Build history of the part. All positions in model axes, mm. A direction names the side the tool comes from. Give positions to 0.01 mm unless a question says otherwise; leave off trailing zeros. Order: outer loops, then holes, each group sorted by start corner. A loop starts at its lowest first (then second) coordinate and runs counter-clockwise, first axis right, second up. Notation, with made-up numbers: (25.25, -13) -> (68.25, -13) arc R31 cw to (68.25, 16) -> close; hole circle Ø3 at (46.5, -31.5). An arc over 180 degrees is marked (long way). One line per question, with ' | ' between items. Start each with the question number.
(1) Drill centre lines: L1, parallel to Y at x = 0, z = 2 (3 decimals); L2, parallel to X at y = 3.5, z = 5.75; L3, parallel to X at y = -6, z = 3.75. Where is each one in solid material? Low to high. Write a range as from..to.
(2) Pull direction X, two halves, no side cores. Call faces 4 (the face through (17, -10.376, 3)), 5 (the face through (48.018, 7.826, 3.451)), 6 (the face through (17, 10.254, 3)), 7 (the face through (34, -15.875, 3)): +X half, -X half, draft (parallel to the pull), parting line (faces both ways), or undercut.
(3) Cut at A-A (x = 0). Give the cut face in (y, z) (3 decimals), then the cut area to 4 significant figures.
(4) Cut at B-B (z = 1.5). Give the cut face in (x, y) (3 decimals), then the cut area to 3 significant figures.
(5) Which spindle directions (+Z, -Z, +X, -X, +Y, -Y) get a long thin tool onto all of the face, cutting with end or side? Do faces 1 (the face through (-17, 10.376, 3)), 2 (the face through (-17, -10.376, 3)), 3 (the face through (47.89, -8.05, 3.45)). Say none if no direction does.
(6) Pin check, flat tips, straight feed: pin 1 Ø3.5 at (x, z) = (-14.5, 4.5) entering from -Y; pin 2 Ø3.5 at (x, z) = (16, 4.5) entering from +Y; pin 3 Ø2 at (x, z) = (-16, 3) entering from +Y; pin 4 Ø10 at (x, y) = (-29, 0) entering from -Z. Stop position of each tip, or through.
(7) Cut at D-D (y = -12). Give the cut face in (x, z).
(8) Cut at C-C (y = 1). Give the cut face in (x, z), then the cut area to 3 significant figures.
from build123d import *

# Parameters (mm, degrees)
F0_R     = 11
F1_DEPTH = 7


with BuildPart() as f1:
    # F0 (on Top) → F1 (new body)
    with BuildSketch(Plane.XY):
        Polygon((-21.865436, -10.375739), (-15.875, 0), (-21.865436, 10.375739), (-25.040436, 15.875), (-43.371307, 15.875), (-52.536742, 0), (-43.371307, -15.875), (-25.040436, -15.875), align=None)
        with Locations((-34.205871, 0)):
            Circle(F0_R, mode=Mode.SUBTRACT)
        with BuildLine():
            ThreePointArc((-12.014977, 10.375739), (-14.878733, 5.535245), (-15.875, 0))
            ThreePointArc((-15.875, 0), (-14.878733, -5.535245), (-12.014977, -10.375739))
            ThreePointArc((-12.014977, -10.375739), (0, -15.875), (12.014977, -10.375739))
            ThreePointArc((12.014977, -10.375739), (14.878733, -5.535245), (15.875, 0))
            ThreePointArc((15.875, 0), (14.906507, 5.460006), (12.1192, 10.25381))
            ThreePointArc((12.1192, 10.25381), (0.080201, 15.874797), (-12.014977, 10.375739))
        make_face()
        Circle(F0_R, mode=Mode.SUBTRACT)
        with BuildLine():
            Line((-21.865436, 10.375739), (-15.875, 0))
            ThreePointArc((-15.875, 0), (-14.878733, 5.535245), (-12.014977, 10.375739))
            Line((-12.014977, 10.375739), (-21.865436, 10.375739))
        make_face()
        with BuildLine():
            ThreePointArc((-12.014977, -10.375739), (-14.878733, -5.535245), (-15.875, 0))
            Line((-15.875, 0), (-21.865436, -10.375739))
            Line((-21.865436, -10.375739), (-12.014977, -10.375739))
        make_face()
        with BuildLine():
            ThreePointArc((15.875, 0), (14.878733, -5.535245), (12.014977, -10.375739))
            Line((12.014977, -10.375739), (21.865436, -10.375739))
            Line((21.865436, -10.375739), (15.875, 0))
        make_face()
        with BuildLine():
            Line((21.79504, 10.25381), (12.1192, 10.25381))
            ThreePointArc((12.1192, 10.25381), (14.906507, 5.460006), (15.875, 0))
            Line((15.875, 0), (21.79504, 10.25381))
        make_face()
        Polygon((21.79504, 10.25381), (15.875, 0), (21.865436, -10.375739), (25.040436, -15.875), (43.371307, -15.875), (52.536742, 0), (43.371307, 15.875), (25.040436, 15.875), align=None)
        with Locations((34.205871, 0)):
            Circle(F0_R, mode=Mode.SUBTRACT)
    extrude(amount=F1_DEPTH)


solid = f1.part
Result set:
1) L1: y = -15.875..-11, 11..15.875 | L2: x = -50.52..-44.63, -23.78..-10.43, 10.43..23.78, 44.63..50.52 | L3: x = -49.07..-43.43, -24.99..-9.22, 9.22..24.99, 43.43..49.07
2) face 4: undercut | face 5: +X half | face 6: undercut | face 7: draft
3) outline: (-15.875, 0) -> (-11, 0) -> (-11, 7) -> (-15.875, 7) -> close; (11, 0) -> (15.875, 0) -> (15.875, 7) -> (11, 7) -> close | area: 68.25 mm2
4) outline: (-52.537, 0) -> (-43.371, -15.875) -> (-25.04, -15.875) -> (-21.865, -10.376) -> (-12.015, -10.376) arc R15.875 ccw to (12.015, -10.376) -> (21.865, -10.376) -> (25.04, -15.875) -> (43.371, -15.875) -> (52.537, 0) -> (43.371, 15.875) -> (25.04, 15.875) -> (21.795, 10.254) -> (12.119, 10.254) arc R15.875 ccw to (-12.015, 10.376) -> (-21.865, 10.376) -> (-25.04, 15.875) -> (-43.371, 15.875) -> close; hole circle Ø22 at (-34.206, 0); hole circle Ø22 at (0, 0); hole circle Ø22 at (34.206, 0) | area: 1,570 mm2
5) face 1: +Z, -Z, +Y | face 2: +Z, -Z, -Y | face 3: +Z, -Z, +X, -Y
6) pin 1: stops at y = -10.38 | pin 2: stops at y = 10.25 | pin 3: stops at y = 10.38 | pin 4: passes through
7) outline: (-45.61, 0) -> (-22.8, 0) -> (-22.8, 7) -> (-45.61, 7) -> close; (-10.39, 0) -> (10.39, 0) -> (10.39, 7) -> (-10.39, 7) -> close; (22.8, 0) -> (45.61, 0) -> (45.61, 7) -> (22.8, 7) -> close
8) outline: (-51.96, 0) -> (-45.16, 0) -> (-45.16, 7) -> (-51.96, 7) -> close; (-23.25, 0) -> (-10.95, 0) -> (-10.95, 7) -> (-23.25, 7) -> close; (10.95, 0) -> (23.25, 0) -> (23.25, 7) -> (10.95, 7) -> close; (45.16, 0) -> (51.96, 0) -> (51.96, 7) -> (45.16, 7) -> close | area: 267 mm2
